```python
from build123d import *

# Parameters (mm, degrees)
SKETCH1_W           = 45
SKETCH1_H           = 130
SKETCH1_R           = 1.6
SKETCH1_R_2         = 1.2
BOSS_EXTRUDE1_DEPTH = 8
FILLET1_R           = 3


with BuildPart() as part:
    # Sketch1 → Boss-Extrude1 (new body)
    with BuildSketch(Plane(origin=(0, 0, 0), x_dir=(1, 0, 0), z_dir=(0, 1, 0))):
        with Locations((22.5, 65)):
            Rectangle(SKETCH1_W, SKETCH1_H)
        with Locations(Location((10, 97.825, 0), (0, 0, 270))):
            Circle(SKETCH1_R, mode=Mode.SUBTRACT)
        with Locations(Location((10, 32.175, 0), (0, 0, 270))):
            Circle(SKETCH1_R, mode=Mode.SUBTRACT)
        with Locations(Location((37, 97.825, 0), (0, 0, 270))):
            Circle(SKETCH1_R_2, mode=Mode.SUBTRACT)
        with Locations(Location((37, 32.175, 0), (0, 0, 270))):
            Circle(SKETCH1_R_2, mode=Mode.SUBTRACT)
        with Locations(Location((22.5, 8, 0), (0, 0, 270))):
            Circle(SKETCH1_R_2, mode=Mode.SUBTRACT)
        with Locations(Location((22.5, 122, 0), (0, 0, 270))):
            Circle(SKETCH1_R_2, mode=Mode.SUBTRACT)
    extrude(amount=BOSS_EXTRUDE1_DEPTH)

    # Fillet1
    fillet1_edges = [part.edges().sort_by_distance(p)[0] for p in [
        (0, 4, 0),
        (0, 4, -130),
        (45, 4, -130),
        (45, 4, 0),
    ]]
    fillet(fillet1_edges, radius=FILLET1_R)


solid = part.part
```
Geometry: final body of the model. Coordinates: model frame, mm. Round coordinates to 2 decimals unless told otherwise and drop trailing zeros. Loops run counter-clockwise (first coordinate to the right, second up) from the corner with the lowest first, then second, coordinate; pieces in that order, holes last. Notation, with made-up numbers: (3, 43.25) -> (22, 43.25) arc R24 ccw to (22, 61.25) -> close; hole circle Ø9 at (85.25, -22.5). An arc over 180 degrees is marked (long way). Use one line per item in the form item = value. Start each with the question number.
1) Draft query along Z for faces 1 (the cylindrical face through (0.86, 4.06, -129.1)), 2 (the cylindrical face through (21.33, 3.94, -8.26)), 3 (the cylindrical face through (38.19, 3.94, -32.33)), 4 (the flat face through (22, 8, -66)). Return one class per face: released by +Z, released by -Z, zero draft, split by the parting line, or undercut.
2) Section C-C on x = 37. Output: boundary loops of the cut face in (y, z) (3 decimals), then the cut area to 3 significant figures.
3) Section B-B on x = 10. Output: boundary loops of the cut face in (y, z) (3 decimals).
4) Line query: L1, parallel to X at y = 5.5, z = -122; L2, parallel to X at y = 1, z = -123. Output: solid intervals per line, ascending.
5) Section A-A on z = -8. Output: boundary loops of the cut face in (x, y).
6) First-contact query: P1, Ø1.4, axis at x = 22.5, z = -8, coming from the -Y side. Flat tip, straight axial feed; report the tip coordinate or a pass-through.
Response:
q1.face_1 = released by -Z
q1.face_2 = undercut
q1.face_3 = undercut
q1.face_4 = zero draft
q2.outline = (0, -130) -> (8, -130) -> (8, -99.025) -> (0, -99.025) -> close; (0, -96.625) -> (8, -96.625) -> (8, -33.375) -> (0, -33.375) -> close; (0, -30.975) -> (8, -30.975) -> (8, 0) -> (0, 0) -> close
q2.area = 1,000 mm^2
q3.outline = (0, -130) -> (8, -130) -> (8, -99.425) -> (0, -99.425) -> close; (0, -96.225) -> (8, -96.225) -> (8, -33.775) -> (0, -33.775) -> close; (0, -30.575) -> (8, -30.575) -> (8, 0) -> (0, 0) -> close
q4.L1 = 0 to 21.3, 23.7 to 45
q4.L2 = 0 to 21.84, 23.16 to 45
q5.outline = (0, 0) -> (21.3, 0) -> (21.3, 8) -> (0, 8) -> close; (23.7, 0) -> (45, 0) -> (45, 8) -> (23.7, 8) -> close
q6.P1 = through
